Source: three-view drawing plus pictorial views. Frame: mm from the lowest corner of the part. A direction names the side the tool comes from. Give positions to 0.01 mm unless a question says otherwise; leave off trailing zeros. Loops run counter-clockwise (first coordinate to the right, second up) from the corner with the lowest first, then second, coordinate; pieces in that order, holes last.
1. Section D-D, the plane x = 10. Output: boundary loops of the cut face in (y, z), then the cut area to 3 significant figures.
2. Draft query along Y for the marked faces 3, 4, 5 and 6. Return one class per face: +Y half, -Y half, draft (parallel to the pull), parting line (faces both ways), or undercut.
3. Material intervals for line 1 along Z through (x, y) = (6.5, 47.05); line 2 along Y through (x, z) = (10, 1.8); line 3 along Y through (x, z) = (34, 1), sorted ascending.
4. Section C-C, the plane y = 26. Output: boundary loops of the cut face in (x, z), then the cut area to 3 significant figures.
5. Section A-A, the plane x = 50. Output: boundary loops of the cut face in (y, z).
6. First-contact query: P1, Ø5, axis at x = 13.5, y = 24.5, coming from the +Z side; P2, Ø10.5, axis at x = 50, z = 34, coming from the -Y side; P3, Ø12, axis at x = 42.5, y = 39.5, coming from the -Z side. Flat tips, straight axial feed; report the tip coordinate or a pass-through.
7. Access query for the marked faces 1 and 2. Directions: +Z, -Z, +X, -X, +Y, -Y. A direction counts if a zero-diameter tool reaches every point of the face in a straight line with its end or side. Return the directions, or none.
8. Section B-B, the plane z = 15. Output: boundary loops of the cut face in (x, y), then the cut area to 3 significant figures.
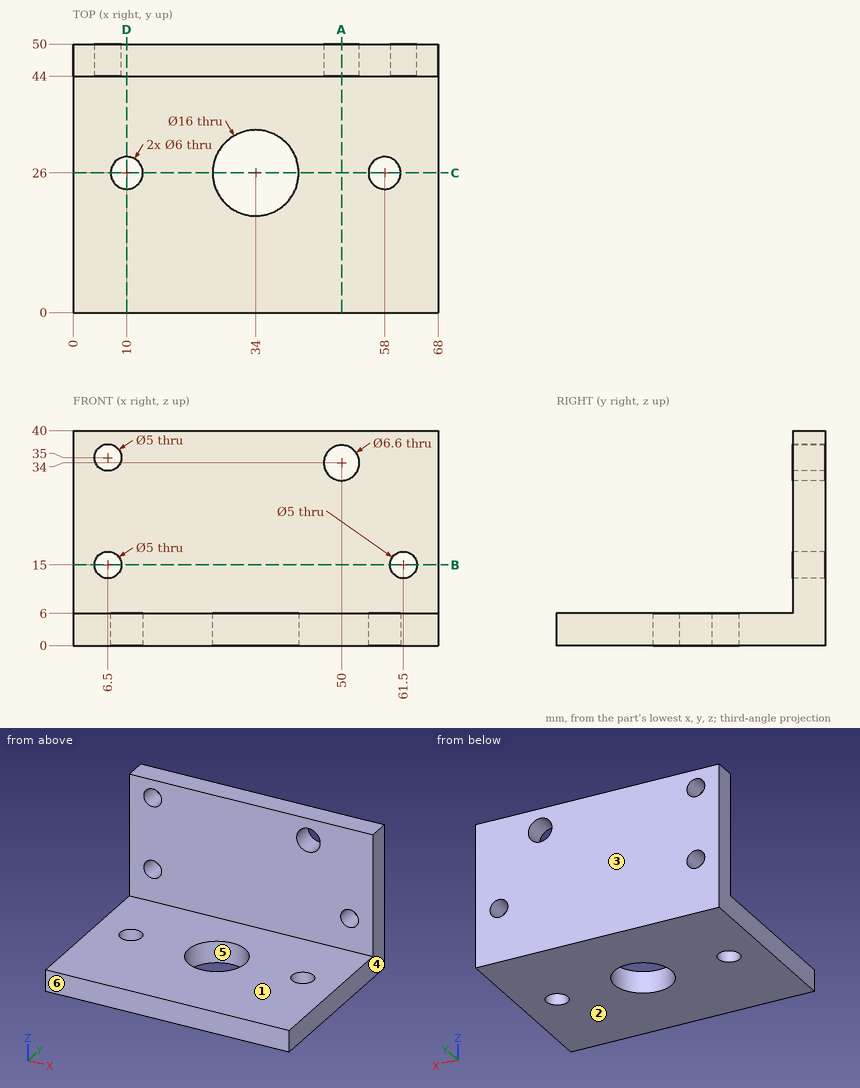
Answers below:
1. outline: (0, 0) - (23, 0) - (23, 6) - (0, 6) - close; (29, 0) - (50, 0) - (50, 40) - (44, 40) - (44, 6) - (29, 6) - close
1. area: 468 mm2
2. face 3: +Y half
2. face 4: draft
2. face 5: undercut
2. face 6: -Y half
3. line 1: z = 0 to 12.5, 17.5 to 32.5, 37.5 to 40
3. line 2: y = 0 to 23, 29 to 50
3. line 3: y = 0 to 18, 34 to 50
4. outline: (0, 0) - (7, 0) - (7, 6) - (0, 6) - close; (13, 0) - (26, 0) - (26, 6) - (13, 6) - close; (42, 0) - (55, 0) - (55, 6) - (42, 6) - close; (61, 0) - (68, 0) - (68, 6) - (61, 6) - close
4. area: 240 mm2
5. outline: (0, 0) - (50, 0) - (50, 30.7) - (44, 30.7) - (44, 6) - (0, 6) - close; (44, 37.3) - (50, 37.3) - (50, 40) - (44, 40) - close
6. P1: stops at z = 6
6. P2: stops at y = 44
6. P3: stops at z = 0
7. face 1: +Z, +X, -X, -Y
7. face 2: -Z, +X, -X, +Y, -Y
8. outline: (0, 44) - (4, 44) - (4, 50) - (0, 50) - close; (9, 44) - (59, 44) - (59, 50) - (9, 50) - close; (64, 44) - (68, 44) - (68, 50) - (64, 50) - close
8. area: 348 mm2
